Model file for the job. Use its own axes, mm. Give positions to 0.01 mm unless a question says otherwise; leave off trailing zeros. Loops run counter-clockwise (first coordinate to the right, second up) from the corner with the lowest first, then second, coordinate; pieces in that order, holes last. Notation, with made-up numbers: (-28.75, -28) - (-16.75, -28) arc R25 cw to (-16.75, -4) - close; hole circle Ø9 at (-28.5, -21.5). An arc over 180 degrees is marked (long way). Answer as CSV lines item,"result". Start each with the question number.
Item 1: Saw through at A-A on z = 25.4. Give the cut face in (x, y), plus the area to 3 significant figures.
Item 2: Pin check, flat tips, straight feed: pin 1 (1.5 mm diameter, centred on x = 6, z = -13.5, fed in from -Y); pin 2 (15 mm diameter, centred on x = 9.525, z = -25.4, fed in from -Y). Stop position of each tip, or through.
Item 3: Saw through at B-B on x = 0. Give the cut face in (y, z).
Item 4: Saw through at C-C on x = 14. Give the cut face in (y, z).
Item 5: Drill centre lines: L1, parallel to Z at x = 9.5, y = 3; L2, parallel to X at y = 3.5, z = 25.4; L3, parallel to X at y = 2.25, z = -25.4 (3 decimals). Where is each one in solid material? Low to high. Write a range as from..to.
Item 6: Saw through at D-D on y = 1.25. Give the cut face in (x, z) (3 decimals).
Autodesk Fusion 360 part; units mm, degrees
sketch "Sketch1" plane through (0, 0, 0) normal (0, 1, 0) x (1, 0, 0)
  line L0 (-6.35, -50.8) -> (25.4, -50.8)
  line L1 (25.4, -50.8) -> (25.4, 50.8)
  line L2 (25.4, 50.8) -> (-6.35, 50.8)
  line L3 (-6.35, 50.8) -> (-6.35, -50.8)
  dimension "d6" = 31.75
  dimension "d7" = 101.6
extrude "Extrude1" add sketch "Sketch1" along normal blind 6.35
hole "Hole1" at (9.525, 0, 25.4) direction (0, 1, 0) diameter 15.9004 depth 12.7 tip angle 118
hole "Hole2" at (9.525, 0, -25.4) direction (0, 1, 0) diameter 25.4 depth 12.7 tip angle 118
fillet "Fillet1" radius 7.62 1 edges at (25.4, 3.175, 50.8)
fillet "Fillet2" radius 7.62 1 edges at (-6.35, 3.175, 50.8)
fillet "Fillet3" radius 7.62 1 edges at (25.4, 3.175, -50.8)
fillet "Fillet4" radius 7.62 1 edges at (-6.35, 3.175, -50.8)
equation "Fit_Height = 4.00 in"
equation "Fit_Length = 1.25 in"
equation "Fit_Width = 0.25 in"
equation "Hole_D1 = 0.626 in"
equation "Hole_D2 = 1.00 in"
equation "d6 = Fit_Length"
equation "d7 = Fit_Height"
equation "d8 = Fit_Width"
equation "d11 = Hole_D1"
equation "d16 = Hole_D2"
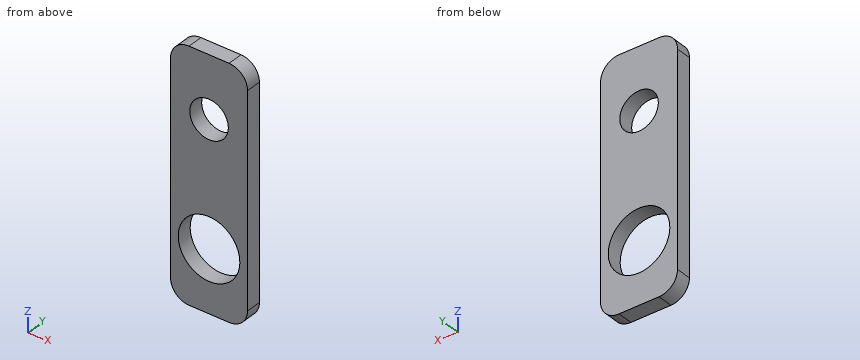
Responses:
1,outline,"(-6.35, 0) - (1.57, 0) - (1.57, 6.35) - (-6.35, 6.35) - close; (17.48, 0) - (25.4, 0) - (25.4, 6.35) - (17.48, 6.35) - close"
1,area,"101 mm2"
2,pin 1,"y = 0"
2,pin 2,"through"
3,outline,"(0, -50.69) - (6.35, -50.69) - (6.35, -33.8) - (0, -33.8) - close; (0, -17) - (6.35, -17) - (6.35, 50.69) - (0, 50.69) - close"
4,outline,"(0, -50.8) - (6.35, -50.8) - (6.35, -37.29) - (0, -37.29) - close; (0, -13.51) - (6.35, -13.51) - (6.35, 18.83) - (0, 18.83) - close; (0, 31.97) - (6.35, 31.97) - (6.35, 50.8) - (0, 50.8) - close"
5,L1,"-50.8..-38.1, -12.7..17.45, 33.35..50.8"
5,L2,"-6.35..1.57, 17.48..25.4"
5,L3,"-6.35..-3.175, 22.225..25.4"
6,outline,"(-6.35, -43.18) arc R7.62 ccw to (1.27, -50.8) - (17.78, -50.8) arc R7.62 ccw to (25.4, -43.18) - (25.4, 43.18) arc R7.62 ccw to (17.78, 50.8) - (1.27, 50.8) arc R7.62 ccw to (-6.35, 43.18) - close; hole circle Ø25.4 at (9.525, -25.4); hole circle Ø15.9 at (9.525, 25.4)"
